```python
from build123d import *

# Parameters (mm, degrees)
F0_W          = 203.2
F0_H          = 3.175
F1_DEPTH      = 25.4
F2_R          = 1.5875
F3_DEPTH      = 25.4
F4_R          = 12.7
F5_DEPTH      = 101.6
F6_R          = 10.16
F7_R          = 2.54
F8_DEPTH      = 254
F9_W          = 63.5
F9_H          = 4.572
F10_DEPTH     = 25.4
F11_W         = 203.2
F11_H         = 25.4
F12_DEPTH     = 3.175
F13_W         = 50.8
F13_H         = 25.4
F14_DEPTH     = 12.7
F15_DEPTH     = 12.7
F16_R         = 5.08
F17_T1_DEPTH  = 15.24
F17_S5_W      = 5.08
F17_S5_H      = 5.08
F17_T6_DEPTH  = 5.08
F17_S11_W     = 5.08
F17_S11_H     = 5.08
F17_T12_DEPTH = 5.08
F17_S17_W     = 5.08
F17_S17_H     = 5.08
F17_T18_DEPTH = 5.08
F17_S23_W     = 5.08
F17_S23_H     = 5.08
F17_T24_DEPTH = 5.08


# Not quite as in the source:
# - a fillet or chamfer that OpenCascade refuses, or shapes differently, is made with other operations: its cross-section is extruded or revolved along the edge and cut away or added


with BuildPart() as f1:
    # F0 (on Front) → F1 (new body)
    with BuildSketch(Plane.XZ):
        with Locations((101.6, 1.5875)):
            Rectangle(F0_W, F0_H)
    extrude(amount=F1_DEPTH)

    # F2 (on face) → F3 (cut)
    with BuildSketch(Plane.XY.offset(3.175)):
        with Locations((12.7, -19.05)):
            Circle(F2_R)
        with Locations((12.7, -6.35)):
            Circle(F2_R)
        with Locations((31.75, -6.35)):
            Circle(F2_R)
        with Locations((31.75, -19.05)):
            Circle(F2_R)
    extrude(amount=-F3_DEPTH, mode=Mode.SUBTRACT)

    # F4 (on face) → F5 (join)
    with BuildSketch(Plane(origin=(0, 0, 0), x_dir=(1, 0, 0), z_dir=(0, 0, -1))):
        with Locations((177.8, 12.7)):
            Circle(F4_R)
    extrude(amount=F5_DEPTH)

    # F6
    f6_edges = [f1.edges().sort_by_distance(p)[0] for p in [
        (165.1, -12.7, -101.6),
    ]]
    fillet(f6_edges, radius=F6_R)

    # F7 (on face) → F8 (cut)
    with BuildSketch(Plane(origin=(0, 0, -101.6), x_dir=(1, 0, 0), z_dir=(0, 0, -1))):
        with Locations((177.8, 12.7)):
            Circle(F7_R)
    extrude(amount=-F8_DEPTH, mode=Mode.SUBTRACT)

    # F9 (on face) → F10 (cut)
    with BuildSketch(Plane.XY.offset(3.175)):
        with Locations((31.75, -12.7)):
            Rectangle(F9_W, F9_H)
    extrude(amount=-F10_DEPTH, mode=Mode.SUBTRACT)

    # F11 (on face) → F12 (join)
    with BuildSketch(Plane.XY.offset(3.175)):
        with Locations((304.8, -12.7)):
            Rectangle(F11_W, F11_H)
    extrude(amount=-F12_DEPTH)

    # F13 (on face) → F14 (join)
    with BuildSketch(Plane.XY.offset(3.175)):
        with Locations((381, -12.7)):
            Rectangle(F13_W, F13_H)
    extrude(amount=F14_DEPTH)

    # F13 (on face) → F15 (join)
    with BuildSketch(Plane.XY.offset(3.175)):
        with Locations((381, -12.7)):
            Rectangle(F13_W, F13_H)
    extrude(amount=-F15_DEPTH)

    # F16
    f16_edges = [f1.edges().sort_by_distance(p)[0] for p in [
        (406.4, -12.7, 15.875),
        (406.4, -12.7, -9.525),
        (355.6, -12.7, 15.875),
        (355.6, -12.7, -9.525),
        (381, -25.4, 15.875),
        (381, -25.4, -9.525),
        (381, 0, 15.875),
        (381, 0, -9.525),
    ]]
    fillet(f16_edges, radius=F16_R)

    # F17: fillet of radius 5.08 on 2 edges, made by hand

    # F17_s2 → F17_t1 (cut)
    with BuildSketch(Plane.XY.offset(-4.445)):
        with BuildLine():
            ThreePointArc((401.32, 0), (404.9121024484, -1.4878975516), (406.4, -5.08))
            Line((406.4, -5.08), (406.4, 0))
            Line((406.4, 0), (401.32, 0))
        make_face()
        with BuildLine():
            ThreePointArc((401.32, -25.4), (404.9121024484, -23.9121024484), (406.4, -20.32))
            Line((406.4, -20.32), (406.4, -25.4))
            Line((406.4, -25.4), (401.32, -25.4))
        make_face()
    extrude(amount=F17_T1_DEPTH, mode=Mode.SUBTRACT)


with BuildPart() as f17_tool4:
    # F17_s5 → F17_t6 (new body)
    with BuildSketch(Plane.XZ.offset(20.32)):
        with Locations((403.86, 13.335)):
            Rectangle(F17_S5_W, F17_S5_H)
    extrude(amount=F17_T6_DEPTH)

    # F17_s7 → F17_t8 (revolve, cut)
    with BuildSketch(Plane(origin=(401.32, -20.32, 10.795), x_dir=(-0.7071067812, 0, -0.7071067812), z_dir=(-0.7071067812, 0, 0.7071067812))):
        with BuildLine():
            ThreePointArc((0, -5.08), (5.08, 0), (0, 5.08))
            Line((0, 5.08), (0, -5.08))
        make_face()
    revolve(axis=Axis((401.32, -20.32, 10.795), (0, -1, 0)), mode=Mode.SUBTRACT)


with BuildPart() as f1_1:
    add(f1.part)

    # F17_t3: cut F17_tool4
    add(f17_tool4.part, mode=Mode.SUBTRACT)


with BuildPart() as f17_tool10:
    # F17_s11 → F17_t12 (new body)
    with BuildSketch(Plane.XZ.offset(5.08)):
        with Locations((403.86, 13.335)):
            Rectangle(F17_S11_W, F17_S11_H)
    extrude(amount=-F17_T12_DEPTH)

    # F17_s13 → F17_t14 (revolve, cut)
    with BuildSketch(Plane(origin=(401.32, -5.08, 10.795), x_dir=(-0.7071067812, 0, -0.7071067812), z_dir=(0.7071067812, 0, -0.7071067812))):
        with BuildLine():
            ThreePointArc((0, -5.08), (5.08, 0), (0, 5.08))
            Line((0, 5.08), (0, -5.08))
        make_face()
    revolve(axis=Axis((401.32, -5.08, 10.795), (0, 1, 0)), mode=Mode.SUBTRACT)


with BuildPart() as f1_2:
    add(f1_1.part)

    # F17_t9: cut F17_tool10
    add(f17_tool10.part, mode=Mode.SUBTRACT)


with BuildPart() as f17_tool16:
    # F17_s17 → F17_t18 (new body)
    with BuildSketch(Plane.XZ.offset(5.08)):
        with Locations((403.86, -6.985)):
            Rectangle(F17_S17_W, F17_S17_H)
    extrude(amount=-F17_T18_DEPTH)

    # F17_s19 → F17_t20 (revolve, cut)
    with BuildSketch(Plane(origin=(401.32, -5.08, -4.445), x_dir=(-0.7071067812, 0, 0.7071067812), z_dir=(-0.7071067812, 0, -0.7071067812))):
        with BuildLine():
            ThreePointArc((0, -5.08), (5.08, 0), (0, 5.08))
            Line((0, 5.08), (0, -5.08))
        make_face()
    revolve(axis=Axis((401.32, -5.08, -4.445), (0, 1, 0)), mode=Mode.SUBTRACT)


with BuildPart() as f1_3:
    add(f1_2.part)

    # F17_t15: cut F17_tool16
    add(f17_tool16.part, mode=Mode.SUBTRACT)


with BuildPart() as f17_tool22:
    # F17_s23 → F17_t24 (new body)
    with BuildSketch(Plane.XZ.offset(20.32)):
        with Locations((403.86, -6.985)):
            Rectangle(F17_S23_W, F17_S23_H)
    extrude(amount=F17_T24_DEPTH)

    # F17_s25 → F17_t26 (revolve, cut)
    with BuildSketch(Plane(origin=(401.32, -20.32, -4.445), x_dir=(-0.7071067812, 0, 0.7071067812), z_dir=(0.7071067812, 0, 0.7071067812))):
        with BuildLine():
            ThreePointArc((0, -5.08), (5.08, 0), (0, 5.08))
            Line((0, 5.08), (0, -5.08))
        make_face()
    revolve(axis=Axis((401.32, -20.32, -4.445), (0, -1, 0)), mode=Mode.SUBTRACT)


with BuildPart() as f1_4:
    add(f1_3.part)

    # F17_t21: cut F17_tool22
    add(f17_tool22.part, mode=Mode.SUBTRACT)


solid = f1_4.part
```
Can you work these out from the model? Positions are in its coordinate system, mm. A direction names the side the tool comes from. Coordinates: 2 decimals unless noted, no trailing zeros. Loops run counter-clockwise (first coordinate to the right, second up) from the corner with the lowest first, then second, coordinate; pieces in that order, holes last.
1) Imagine slicing it at D-D on x = 309. List the corners of the cut face in (y, z) for me (3 decimals), plus the area to 3 significant figures.
2) Imagine slicing it at B-B on z = -68.5. List the corners of the cut face in (x, y) for me.
3) Which directions (+Z, -Z, +X, -X, +Y, -Y) give clear straight access to the entire face, cutting with the end or side of a thin tool? Please do faces 1 (the flat face through (175, -15, 3.175)), 2 (the flat face through (244, 0, 2)), 3 (the cylindrical face through (168.44, -21.283, -45.08)).
4) Imagine slicing it at C-C on x = 375.5. List the corners of the cut face in (y, z) for me (3 decimals), plus the area to 3 significant figures.
5) For pin 1 (1 mm diameter, centred on y = -14, z = 1, fed in from -X); pin 2 (3 mm diameter, centred on x = 218, z = 3.5, fed in from +Y); pin 3 (3 mm diameter, centred on x = 149, y = -3.5, fed in from -Z); pin 4 (1.3 mm diameter, centred on y = -7.5, z = -2, fed in from -X), each with a flat end and sliding along its axis, tell me the tip position at first contact or that it passes through.
6) Thinking about a two-plate mould opening in X: for faces 4 (the flat face through (355.6, -13, 7)), 5 (the flat face through (381, -13, -9.525)), 6 (the flat face through (265, -13, 0)), 7 (the flat face through (406.4, -13, 3)), which applies, pulls with the +X half, pulls with the -X half, needs draft (parallel to the pull), parting line crosses it, or undercut?
7) I need wall thicknesses on probe 1 along X at (y, z) = (-12.7, -73.5); probe 2 along Z at (x, y) = (113, -20.25) (3 decimals); probe 3 along Y at (x, z) = (12, 1). Which ranges of each line are inside material? Lowest first, please.
8) Imagine slicing it at A-A on x = 47. List the corners of the cut face in (y, z) for me (3 decimals), plus the area to 3 significant figures.
Completed:
1. outline: (-25.4, 0) - (0, 0) - (0, 3.175) - (-25.4, 3.175) - close
1. area: 80.6 mm2
2. outline: circle Ø25.4 at (177.8, -12.7); hole circle Ø5.08 at (177.8, -12.7)
3. face 1: +Z, -X, +Y, -Y
3. face 2: +Z, -Z, +X, -X, +Y
3. face 3: -Z
4. outline: (-25.4, -4.445) arc R5.08 ccw to (-20.32, -9.525) - (-5.08, -9.525) arc R5.08 ccw to (0, -4.445) - (0, 10.795) arc R5.08 ccw to (-5.08, 15.875) - (-20.32, 15.875) arc R5.08 ccw to (-25.4, 10.795) - close
4. area: 623 mm2
5. pin 1: stops at x = 63.5
5. pin 2: stops at y = 0
5. pin 3: stops at z = 0
5. pin 4: stops at x = 165.94
6. face 4: pulls with the -X half
6. face 5: needs draft
6. face 6: undercut
6. face 7: pulls with the +X half
7. probe 1: x = 165.1 to 175.26, 180.34 to 190.5
7. probe 2: z = 0 to 3.175
7. probe 3: y = -25.4 to -20.47, -17.63 to -14.99, -10.41 to -7.77, -4.93 to 0
8. outline: (-25.4, 0) - (-14.986, 0) - (-14.986, 3.175) - (-25.4, 3.175) - close; (-10.414, 0) - (0, 0) - (0, 3.175) - (-10.414, 3.175) - close
8. area: 66.1 mm2
